Here's how the part is built. I have some questions about the finished solid (model axes, mm). Round coordinates to 2 decimals unless told otherwise and drop trailing zeros. Order: outer loops, then holes, each group sorted by start corner. A loop starts at its lowest first (then second) coordinate and runs counter-clockwise, first axis right, second up. Notation, with made-up numbers: M 65.5,23.5 L 88.5,23.5 A8 ccw 88.5,28.5 Z; hole C -20,41 d5. An arc over 180 degrees is marked long. Write each question's results on one line, items separated by ' | '. Start each with the question number.
Solid Edge part; units mm, degrees
sketch "Sketch1" plane through (0, 0, 0) normal (0, 0, 1) x (1, 0, 0)
  line L0 (0, 0) -> (20, 0)
  line L1 (20, 0) -> (20, 50)
  circle A0 centre (21, 25) radius 14.3
  line L2 (20, 50) -> (0, 50)
  line L3 (0, 50) -> (0, 0)
extrude "Protrusion1" add sketch "Sketch1" along normal blind 15
hole "Bohrung_1" at (20, 5.3675, 7.5) direction (-1, 0, 0) diameter 4.5 end through all
hole "Hole1" at (20, 44.6325, 7.5) direction (-1, 0, 0) diameter 4.5 end through all
fillet "Verrundung_2" radius 0.5 6 edges at (0, 50, 7.5) (0, 0, 7.5) (20, 0, 7.5) (20, 10.735, 7.5) (20, 39.265, 7.5) (20, 50, 7.5)
(1) I want a section at B-B on z = 7.5. Write out the boundary of the cut face in (x, y).
(2) I want a section at C-C on y = 44. Write out the boundary of the cut face in (x, z), and give its area (3 significant figures).
(3) Please list where these lines run through material, in increasing order: line 1 (Y direction, x = 6, z = 7.5); line 2 (Y direction, x = 12.75, z = 7.5); line 3 (Y direction, x = 5.75, z = 5.75).
(4) I want a section at A-A on x = 7.75. Write out the boundary of the cut face in (y, z), and give its area (3 significant figures).
(5) I'm going to push flat-ended pins straight in: pin 1 Ø6 at (y, z) = (28.5, 6) entering from +X; pin 2 Ø1 at (y, z) = (37.5, 5) entering from +X. Where does each tip first touch, or does it pass through?
(6) If we mould it in two halves opening along Z, with no side actions, what happens to faces 1 (the cylindrical face through (10.14, 43.263, 9.286)), 2 (the flat face through (20, 3, 9)), 3 (the cylindrical face through (10.14, 3.998, 9.286)), 4 (the flat face through (5, 25, 15))? For each: pulls with the +Z half, pulls with the -Z half, needs draft (parallel to the pull), parting line crosses it, or undercut.
(7) I want a section at D-D on z = 10.25. Write out the boundary of the cut face in (x, y).
Solutions:
1) outline: M 0,0.5 A0.5 ccw 0.5,0 L 19.5,0 A0.5 ccw 20,0.5 L 20,3.12 L 0,3.12 Z; M 0,7.62 L 20,7.62 L 20,10.28 A0.5 ccw 19.55,10.77 A14.3 cw 19.55,39.23 A0.5 ccw 20,39.72 L 20,42.38 L 0,42.38 Z; M 0,46.88 L 20,46.88 L 20,49.5 A0.5 ccw 19.5,50 L 0.5,50 A0.5 ccw 0,49.5 Z
2) outline: M 0,0 L 20,0 L 20,5.34 L 0,5.34 Z; M 0,9.66 L 20,9.66 L 20,15 L 0,15 Z | area: 214 mm^2
3) line 1: 0 to 3.12, 7.62 to 42.38, 46.88 to 50 | line 2: 0 to 3.12, 7.62 to 13.32, 36.68 to 42.38, 46.88 to 50 | line 3: 0 to 3.95, 6.78 to 43.22, 46.05 to 50
4) outline: M 0,0 L 19.62,0 L 19.62,15 L 0,15 Z; M 30.38,0 L 50,0 L 50,15 L 30.38,15 Z; hole C 5.37,7.5 d4.5; hole C 44.63,7.5 d4.5 | area: 557 mm^2
5) pin 1: x = 8.26 | pin 2: x = 15.04
6) face 1: undercut | face 2: needs draft | face 3: undercut | face 4: pulls with the +Z half
7) outline: M 0,0.5 A0.5 ccw 0.5,0 L 19.5,0 A0.5 ccw 20,0.5 L 20,10.28 A0.5 ccw 19.55,10.77 A14.3 cw 19.55,39.23 A0.5 ccw 20,39.72 L 20,49.5 A0.5 ccw 19.5,50 L 0.5,50 A0.5 ccw 0,49.5 Z
